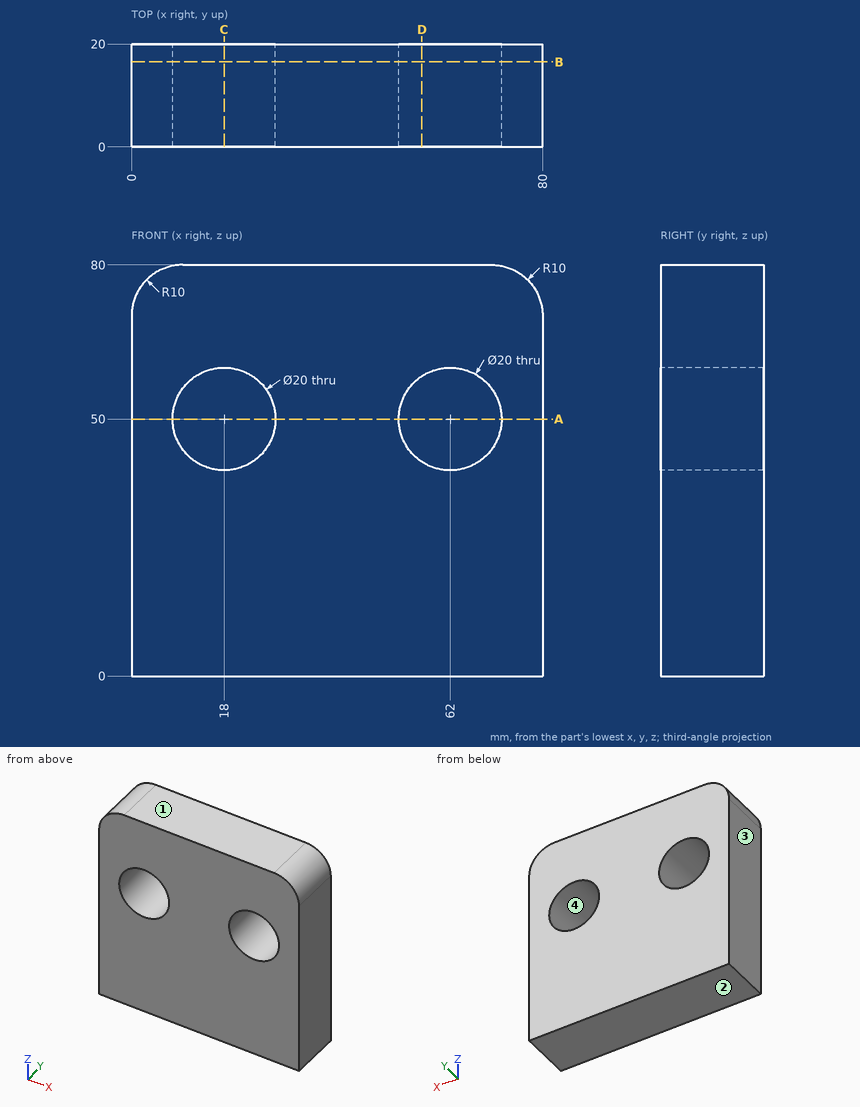
Could you check a few things on this drawing? It's one solid part, dimensions in mm from its lowest x, y, z. Coordinates: 2 decimals unless noted, no trailing zeros. Order: outer loops, then holes, each group sorted by start corner. A loop starts at its lowest first (then second) coordinate and runs counter-clockwise, first axis right, second up.
1. If we section it at C-C (x = 18): Please give me the cut outline in (y, z), then the cut area to 3 significant figures.
2. If we section it at D-D (x = 56.5): Please give me the cut outline in (y, z).
3. Thinking about a two-plate mould opening in Z: for the marked faces 1, 2, 3 and 4, which applies, +Z half, -Z half, draft (parallel to the pull), parting line (faces both ways), or undercut?
4. I need wall thicknesses on line 1 (X direction, y = 10.25, z = 50); line 2 (X direction, y = 5.25, z = 44); line 3 (Z direction, x = 13, y = 11.25). Which ranges of each line are inside material? Lowest first, please.
5. If we section it at A-A (z = 50): Please give me the cut outline in (x, y).
6. I'm going to push flat-ended pins straight in: pin 1 (12 mm diameter, centred on x = 30, z = 40.5, fed in from -Y); pin 2 (12 mm diameter, centred on x = 62, z = 50, fed in from -Y). Where does each tip first touch, or does it pass through?
7. If we section it at B-B (y = 16.5): Please give me the cut outline in (x, z), then the cut area to 3 significant figures.
Entries:
1. outline: (0, 0) - (20, 0) - (20, 40) - (0, 40) - close; (0, 60) - (20, 60) - (20, 80) - (0, 80) - close
1. area: 1,200 mm2
2. outline: (0, 0) - (20, 0) - (20, 41.65) - (0, 41.65) - close; (0, 58.35) - (20, 58.35) - (20, 80) - (0, 80) - close
3. face 1: +Z half
3. face 2: -Z half
3. face 3: draft
3. face 4: undercut
4. line 1: x = 0 to 8, 28 to 52, 72 to 80
4. line 2: x = 0 to 10, 26 to 54, 70 to 80
4. line 3: z = 0 to 41.34, 58.66 to 80
5. outline: (0, 0) - (8, 0) - (8, 20) - (0, 20) - close; (28, 0) - (52, 0) - (52, 20) - (28, 20) - close; (72, 0) - (80, 0) - (80, 20) - (72, 20) - close
6. pin 1: stops at y = 0
6. pin 2: passes through
7. outline: (0, 0) - (80, 0) - (80, 70) arc R10 ccw to (70, 80) - (10, 80) arc R10 ccw to (0, 70) - close; hole circle Ø20 at (18, 50); hole circle Ø20 at (62, 50)
7. area: 5,730 mm2
